Geometry: final body of the model. Coordinates: model frame, mm. A direction names the side the tool comes from. Give positions to 0.01 mm unless a question says otherwise; leave off trailing zeros. Order: outer loops, then holes, each group sorted by start corner. A loop starts at its lowest first (then second) coordinate and runs counter-clockwise, first axis right, second up. Notation, with made-up numbers: (-1.75, 35.5) -> (7.25, 35.5) arc R35 cw to (7.25, 70.5) -> close; hole circle Ø3 at (30.5, 40.25). An arc over 180 degrees is marked (long way). Answer in a Markdown table with one row per item. Add a question column.
Q1. Cut plane C-C on z = 175. Return the cut outline in (x, y), and give its area (3 significant figures).
Q2. Cut plane A-A on y = 13.75. Return the cut outline in (x, z), and give its area (3 significant figures).
Q3. Set-up query: faces 5 (the face through (0, 5, 200)), 6 (the face through (0, 19, 195)), 7 (the face through (2, 5, 173)). Return all of +Z, -Z, +X, -X, +Y, -Y with unobstructed straight access to the full face (end or side cutting, diameter ignored); none if empty.
Q4. Cut plane B-B on x = -0.75. Return the cut outline in (y, z), and give its area (3 significant figures).
Q5. Pull-direction query (X, two-part tool) for faces 1 (the face through (3.76, 14.805, 165.827)), 2 (the face through (0.34, 16.93, 172.37)), 3 (the face through (-2.1, 2.46, 183.42)), 4 (the face through (0, 29.2, 180)); classes: +X half, -X half, draft (parallel to the pull), parting line (faces both ways), or undercut.
Q6. Cut plane D-D on x = 1.25. Return the cut outline in (y, z).
Q7. Contact query for flat-ended pins moving along their axis: P1, Ø4, axis at y = 2, z = 186, coming from the -X side; P2, Ø5, axis at x = 0, z = 175, coming from the -Y side; P3, Ø1, axis at x = 0, y = 26, coming from the +Z side; P4, Ø10, axis at y = 22.5, z = 195, coming from the +X side. Output: stop coordinate, or through.
Q8. Line query: line 1 along Z through (x, y) = (0, 14); line 2 along Z through (x, y) = (-4, 4); line 3 along X through (y, z) = (17.5, 175). Output: solid intervals per line, ascending. Write a range as from..to.
from build123d import *

# Parameters (mm, degrees)
EXTRUDE_590_DEPTH   = 29.2
EXTRUDE_638_DEPTH   = 9.5
FILLET_1_R          = 3
HOLE_WIZARD_M5_1_D  = 5.3
CUT_EXTRUDE_1_DEPTH = 5
CUT_EXTRUDE_2_DEPTH = 0.1


with BuildPart() as part:
    # 草图1 → Extrude 590 (new body)
    with BuildSketch(Plane(origin=(0, 0, 0), x_dir=(1, 0, 0), z_dir=(0, 1, 0))):
        with BuildLine():
            Line((4.608867317, -165), (-4.608867317, -165))
            Line((-4.608867317, -165), (-5.444719551, -194.923972433))
            ThreePointArc((-5.444719551, -194.923972433), (0, -195), (5.444719551, -194.923972433))
            Line((5.444719551, -194.923972433), (4.608867317, -165))
        make_face()
    extrude(amount=EXTRUDE_590_DEPTH)

    # 草图1<3> → Extrude 638 (add)
    with BuildSketch(Plane(origin=(0, 0, 0), x_dir=(1, 0, 0), z_dir=(0, 1, 0))):
        with BuildLine():
            ThreePointArc((5.444719551, -194.923972433), (0, -195), (-5.444719551, -194.923972433))
            Line((-5.444719551, -194.923972433), (-5.584327745, -199.922023008))
            ThreePointArc((-5.584327745, -199.922023008), (0, -200), (5.584327745, -199.922023008))
            Line((5.584327745, -199.922023008), (5.444719551, -194.923972433))
        make_face()
    extrude(amount=EXTRUDE_638_DEPTH)

    # 圆角1
    fillet_1_edges = [part.edges().sort_by_distance(p)[0] for p in [
        (4.608867317, 14.6, 165),
        (0, 0, 165),
        (-4.608867317, 14.6, 165),
    ]]
    fillet(fillet_1_edges, radius=FILLET_1_R)

    # M5 间隙孔1 (through all)
    with Locations(Plane(origin=(0, 29.2, 0), x_dir=(1, 0, 0), z_dir=(0, 1, 0))):
        with Locations((0, -187), (0, -175)):
            Hole(HOLE_WIZARD_M5_1_D / 2)

    # 草图6 → 切除-拉伸1 (cut)
    with BuildSketch(Plane.XZ):
        Polygon((0, 179.792007234), (-4.15, 177.396003617), (-4.15, 172.603996383), (0, 170.207992766), (4.15, 172.603996383), (4.15, 177.396003617), align=None)
        Polygon((0, 191.792007234), (-4.15, 189.396003617), (-4.15, 184.603996383), (0, 182.207992766), (4.15, 184.603996383), (4.15, 189.396003617), align=None)
    extrude(amount=-CUT_EXTRUDE_1_DEPTH, mode=Mode.SUBTRACT)

    # 草图7 → 切除-拉伸2 (cut)
    with BuildSketch(Plane(origin=(0, 0, 0), x_dir=(-0.02792163872356911, 0, -0.9996101150403545), z_dir=(0.9996101150403545, 0, -0.02792163872356911))):
        with BuildLine():
            Line((-172.3983953, 26.892307692), (-172.712497864, 26.892307692))
            add(Edge.make_bspline(
                [(-172.712497864, 26.892307692), (-172.703988313, 26.927540176), (-172.687352838, 26.996416801), (-172.652655264, 27.094824062), (-172.614856009, 27.187947583), (-172.569466905, 27.274043657), (-172.51995815, 27.354842559), (-172.463235429, 27.428511684), (-172.401915706, 27.496924649), (-172.334090757, 27.557637887), (-172.262962095, 27.612615616), (-172.187527476, 27.659490673), (-172.109304582, 27.699814826), (-172.027751449, 27.733035058), (-171.942625277, 27.758060582), (-171.854695654, 27.776217387), (-171.763732154, 27.788008502), (-171.701984563, 27.789159265), (-171.670630877, 27.78974359)],
                knots=[0, 0, 0, 0, 1.162005537, 2.271625781, 3.343758855, 4.383309926, 5.390229558, 6.379919256, 7.361854164, 8.333198761, 9.295911338, 10.242430842, 11.177959212, 12.116337295, 13.062827104, 14.020064771, 14.994644689, 16, 16, 16, 16], degree=3))
            add(Edge.make_bspline(
                [(-171.670630877, 27.78974359), (-171.624948135, 27.788364359), (-171.534579124, 27.785635984), (-171.401816077, 27.760721548), (-171.273789258, 27.721296415), (-171.15190001, 27.666822688), (-171.038681577, 27.599635375), (-170.937945391, 27.519670638), (-170.85105688, 27.428471337), (-170.778162502, 27.327738772), (-170.721087503, 27.220083263), (-170.67900113, 27.109283106), (-170.653379449, 26.995601134), (-170.650058892, 26.918843855), (-170.6483953, 26.880388622)],
                knots=[0, 0, 0, 0, 1.083050992, 2.142477498, 3.193116406, 4.255571735, 5.30263384, 6.308962982, 7.297363603, 8.282367274, 9.249857812, 10.179914175, 11.08814088, 12, 12, 12, 12], degree=3))
            add(Edge.make_bspline(
                [(-170.6483953, 26.880388622), (-170.649558891, 26.843381827), (-170.651835858, 26.770965273), (-170.671169564, 26.665243775), (-170.703705827, 26.565602175), (-170.748775589, 26.471621013), (-170.807117139, 26.383896173), (-170.877789836, 26.302230282), (-170.961292498, 26.226261124), (-171.024571436, 26.182741651), (-171.057149306, 26.160336538)],
                knots=[0, 0, 0, 0, 1.024540389, 2.004866551, 2.965041327, 3.920577974, 4.882998113, 5.874504559, 6.905732034, 8, 8, 8, 8], degree=3))
            add(Edge.make_bspline(
                [(-171.057149306, 26.160336538), (-171.019917552, 26.142358367), (-170.946150678, 26.106738409), (-170.845600148, 26.036882652), (-170.754322273, 25.956226304), (-170.703418554, 25.893283652), (-170.677842415, 25.861658654)],
                knots=[0, 0, 0, 0, 1.015518401, 2.012035669, 3.001164323, 4, 4, 4, 4], degree=3))
            add(Edge.make_bspline(
                [(-170.677842415, 25.861658654), (-170.661001073, 25.838600902), (-170.627594177, 25.792862986), (-170.586358643, 25.71932656), (-170.548949529, 25.644975071), (-170.51979931, 25.567815664), (-170.497225443, 25.488742651), (-170.48108941, 25.407620255), (-170.47106527, 25.324382232), (-170.469629718, 25.268069752), (-170.46890812, 25.239763622)],
                knots=[0, 0, 0, 0, 1.025084078, 2.033381695, 3.024893161, 4.013698104, 4.991890475, 5.976764909, 6.982997093, 8, 8, 8, 8], degree=3))
            add(Edge.make_bspline(
                [(-170.46890812, 25.239763622), (-170.470702634, 25.190753901), (-170.474283216, 25.092965099), (-170.50628729, 24.948490377), (-170.555900531, 24.807264875), (-170.626357467, 24.672190036), (-170.712224976, 24.545809655), (-170.8143823, 24.432733346), (-170.931668708, 24.335534741), (-171.062474357, 24.254324513), (-171.204191486, 24.189406591), (-171.355767078, 24.144349148), (-171.515017132, 24.115003148), (-171.624224429, 24.11185628), (-171.67974546, 24.11025641)],
                knots=[0, 0, 0, 0, 0.955779014, 1.907060117, 2.875433937, 3.871313158, 4.872415639, 5.851225146, 6.836215519, 7.83643374, 8.849228613, 9.86973379, 10.916971861, 12, 12, 12, 12], degree=3))
            add(Edge.make_bspline(
                [(-171.67974546, 24.11025641), (-171.717164761, 24.111124624), (-171.790793466, 24.112832978), (-171.899036964, 24.124511579), (-172.002358663, 24.145841584), (-172.100898261, 24.174544889), (-172.194743298, 24.210936632), (-172.283607403, 24.25625533), (-172.368037296, 24.309566832), (-172.447236247, 24.371500419), (-172.521194815, 24.440781759), (-172.587947539, 24.518640769), (-172.648607332, 24.603638173), (-172.701549971, 24.696761229), (-172.749186924, 24.796806487), (-172.78836788, 24.905054985), (-172.822853449, 25.020539007), (-172.838886913, 25.101016747), (-172.847113249, 25.142307692)],
                knots=[0, 0, 0, 0, 1.048658725, 2.063410685, 3.046034179, 4.001477787, 4.936774919, 5.862367409, 6.792675028, 7.730719943, 8.675894397, 9.627829632, 10.600096036, 11.597688215, 12.626045268, 13.701542398, 14.82072376, 16, 16, 16, 16], degree=3))
            Line((-172.847113249, 25.142307692), (-172.533010685, 25.142307692))
            add(Edge.make_bspline(
                [(-172.533010685, 25.142307692), (-172.524827393, 25.115358679), (-172.508910181, 25.062940507), (-172.481815882, 24.987500202), (-172.45094761, 24.918342149), (-172.417833052, 24.854959027), (-172.383054606, 24.796726624), (-172.344139681, 24.745184755), (-172.303970535, 24.698069553), (-172.273691182, 24.671524941), (-172.258872063, 24.658533654)],
                knots=[0, 0, 0, 0, 1.198163088, 2.33053128, 3.407730985, 4.417276592, 5.372219308, 6.28897303, 7.162600585, 8, 8, 8, 8], degree=3))
            add(Edge.make_bspline(
                [(-172.258872063, 24.658533654), (-172.239275486, 24.64342532), (-172.200142823, 24.613255288), (-172.136374592, 24.57475366), (-172.069309706, 24.541392634), (-171.997495032, 24.515908939), (-171.922480262, 24.494331278), (-171.843052896, 24.480210759), (-171.759913679, 24.470522587), (-171.703145916, 24.469667656), (-171.674136486, 24.469230769)],
                knots=[0, 0, 0, 0, 0.946170439, 1.889420265, 2.845303464, 3.807233317, 4.801018734, 5.828864929, 6.890507805, 8, 8, 8, 8], degree=3))
            add(Edge.make_bspline(
                [(-171.674136486, 24.469230769), (-171.641382983, 24.469846674), (-171.577336336, 24.471051024), (-171.483881477, 24.482126731), (-171.394974029, 24.498257144), (-171.311601104, 24.523170127), (-171.232670596, 24.553950979), (-171.159288947, 24.592599384), (-171.09049284, 24.637944106), (-171.027163435, 24.689483264), (-170.970217928, 24.745904759), (-170.920078414, 24.80491783), (-170.877453753, 24.86627366), (-170.843070175, 24.930311781), (-170.815919624, 24.99676701), (-170.797436424, 25.065825839), (-170.784584909, 25.136923105), (-170.783538296, 25.185252074), (-170.783010685, 25.209615385)],
                knots=[0, 0, 0, 0, 1.217147791, 2.380027433, 3.494444702, 4.572153297, 5.609568379, 6.639424714, 7.649109417, 8.668170816, 9.669597737, 10.625200337, 11.543417969, 12.441394052, 13.322311151, 14.205496177, 15.095365482, 16, 16, 16, 16], degree=3))
            add(Edge.make_bspline(
                [(-170.783010685, 25.209615385), (-170.784540986, 25.242226723), (-170.787593975, 25.307287132), (-170.810902554, 25.403004706), (-170.849241418, 25.495228118), (-170.90291393, 25.582383909), (-170.968249658, 25.66315981), (-171.044614565, 25.735231293), (-171.132642793, 25.794701384), (-171.213662662, 25.83579004), (-171.285427819, 25.863827115), (-171.346843203, 25.88250208), (-171.415599807, 25.898315735), (-171.490866156, 25.913028007), (-171.573209372, 25.925549355), (-171.66253981, 25.935991171), (-171.758875572, 25.944346212), (-171.825566738, 25.948077307), (-171.859933762, 25.95)],
                knots=[0, 0, 0, 0, 1.07054697, 2.135767047, 3.216561865, 4.33974944, 5.486079747, 6.621378074, 7.775625952, 8.963672916, 9.598146892, 10.304877434, 11.070270905, 11.915000392, 12.823868403, 13.805723172, 14.86925407, 16, 16, 16, 16], degree=3))
            Line((-171.859933762, 25.95), (-171.859933762, 26.308974359))
            add(Edge.make_bspline(
                [(-171.859933762, 26.308974359), (-171.816632596, 26.309709163), (-171.731816249, 26.311148463), (-171.607921944, 26.328556473), (-171.489448632, 26.352637101), (-171.37902189, 26.389522293), (-171.278373177, 26.43236259), (-171.191053575, 26.4822148), (-171.118286428, 26.537629549), (-171.060425356, 26.599462158), (-171.016896128, 26.665777206), (-170.98506933, 26.734893864), (-170.966269004, 26.807417924), (-170.963759337, 26.856912592), (-170.962497864, 26.881790865)],
                knots=[0, 0, 0, 0, 1.321986639, 2.589447074, 3.816329219, 5.01088745, 6.139805852, 7.153945165, 8.075214402, 8.924034688, 9.728124013, 10.488707548, 11.240355623, 12, 12, 12, 12], degree=3))
            add(Edge.make_bspline(
                [(-170.962497864, 26.881790865), (-170.962912275, 26.900068611), (-170.963736726, 26.936431318), (-170.974134004, 26.989556386), (-170.989758045, 27.041057332), (-171.011237774, 27.090715142), (-171.039987973, 27.138185416), (-171.074393959, 27.183872865), (-171.11536206, 27.227516644), (-171.162307507, 27.268196964), (-171.212719312, 27.306966201), (-171.267969087, 27.339879838), (-171.326390961, 27.3680249), (-171.388049616, 27.391234402), (-171.453145146, 27.40869369), (-171.521371704, 27.421229532), (-171.592859388, 27.429067187), (-171.64163112, 27.430195602), (-171.666424146, 27.430769231)],
                knots=[0, 0, 0, 0, 0.884392785, 1.759457502, 2.611959086, 3.489218968, 4.37281399, 5.2945488, 6.255912374, 7.266815255, 8.301784654, 9.332968512, 10.37626691, 11.440494194, 12.520033166, 13.637162961, 14.798855837, 16, 16, 16, 16], degree=3))
            add(Edge.make_bspline(
                [(-171.666424146, 27.430769231), (-171.706275814, 27.429377869), (-171.784115391, 27.426660215), (-171.896330307, 27.402857202), (-172.000649641, 27.364879118), (-172.080388308, 27.319546099), (-172.139270882, 27.274795665), (-172.18134782, 27.235713279), (-172.222668331, 27.192280455), (-172.260514008, 27.14182208), (-172.298787984, 27.087755289), (-172.333632546, 27.027331608), (-172.367492238, 26.962127214), (-172.387894788, 26.916031579), (-172.3983953, 26.892307692)],
                knots=[0, 0, 0, 0, 1.472543308, 2.876219568, 4.221790263, 5.565193594, 6.249813518, 6.953379497, 7.687249741, 8.463570142, 9.283606569, 10.136032583, 11.040678096, 12, 12, 12, 12], degree=3))
        make_face()
    extrude(amount=-CUT_EXTRUDE_2_DEPTH, mode=Mode.SUBTRACT)


solid = part.part
Completed:
| question | item | result |
|---|---|---|
| 1 | outline | (-4.89, 0) -> (-4.15, 0) -> (-4.15, 5) -> (-2.65, 5) -> (-2.65, 29.2) -> (-4.89, 29.2) -> close; (2.65, 5) -> (4.15, 5) -> (4.15, 0) -> (4.89, 0) -> (4.89, 29.2) -> (2.65, 29.2) -> close |
| 1 | area | 116 mm² |
| 2 | outline | (-5.44, 194.92) -> (-4.69, 167.92) arc R3 ccw to (-1.69, 165) -> (1.69, 165) arc R3 ccw to (4.69, 167.92) -> (5.44, 194.92) arc R195 ccw to start; hole circle Ø5.3 at (0, 175); hole circle Ø5.3 at (0, 187) |
| 2 | area | 254 mm² |
| 3 | face 5 | +Z, +Y, -Y |
| 3 | face 6 | +Z, +Y |
| 3 | face 7 | -Y |
| 4 | outline | (0, 168) arc R3 ccw to (3, 165) -> (29.2, 165) -> (29.2, 172.46) -> (5, 172.46) -> (5, 170.64) -> (0, 170.64) -> close; (0, 179.36) -> (5, 179.36) -> (5, 177.54) -> (29.2, 177.54) -> (29.2, 184.46) -> (5, 184.46) -> (5, 182.64) -> (0, 182.64) -> close; (0, 191.36) -> (5, 191.36) -> (5, 189.54) -> (29.2, 189.54) -> (29.2, 195) -> (9.5, 195) -> (9.5, 200) -> (0, 200) -> close |
| 4 | area | 588 mm² |
| 5 | face 1 | +X half |
| 5 | face 2 | undercut |
| 5 | face 3 | undercut |
| 5 | face 4 | draft |
| 6 | outline | (0, 168) arc R3 ccw to (3, 165) -> (29.2, 165) -> (29.2, 172.66) -> (5, 172.66) -> (5, 170.93) -> (0, 170.93) -> close; (0, 179.07) -> (5, 179.07) -> (5, 177.34) -> (29.2, 177.34) -> (29.2, 184.66) -> (5, 184.66) -> (5, 182.93) -> (0, 182.93) -> close; (0, 191.07) -> (5, 191.07) -> (5, 189.34) -> (29.2, 189.34) -> (29.2, 195) -> (9.5, 195) -> (9.5, 200) -> (0, 200) -> close |
| 7 | P1 | stops at x = -5.25 |
| 7 | P2 | passes through |
| 7 | P3 | stops at z = 195 |
| 7 | P4 | stops at x = 5.44 |
| 8 | line 1 | z = 165..172.35, 177.65..184.35, 189.65..195 |
| 8 | line 2 | z = 166.08..172.52, 177.48..184.52, 189.48..199.96 |
| 8 | line 3 | x = -4.89..-2.65, 2.65..4.89 |
